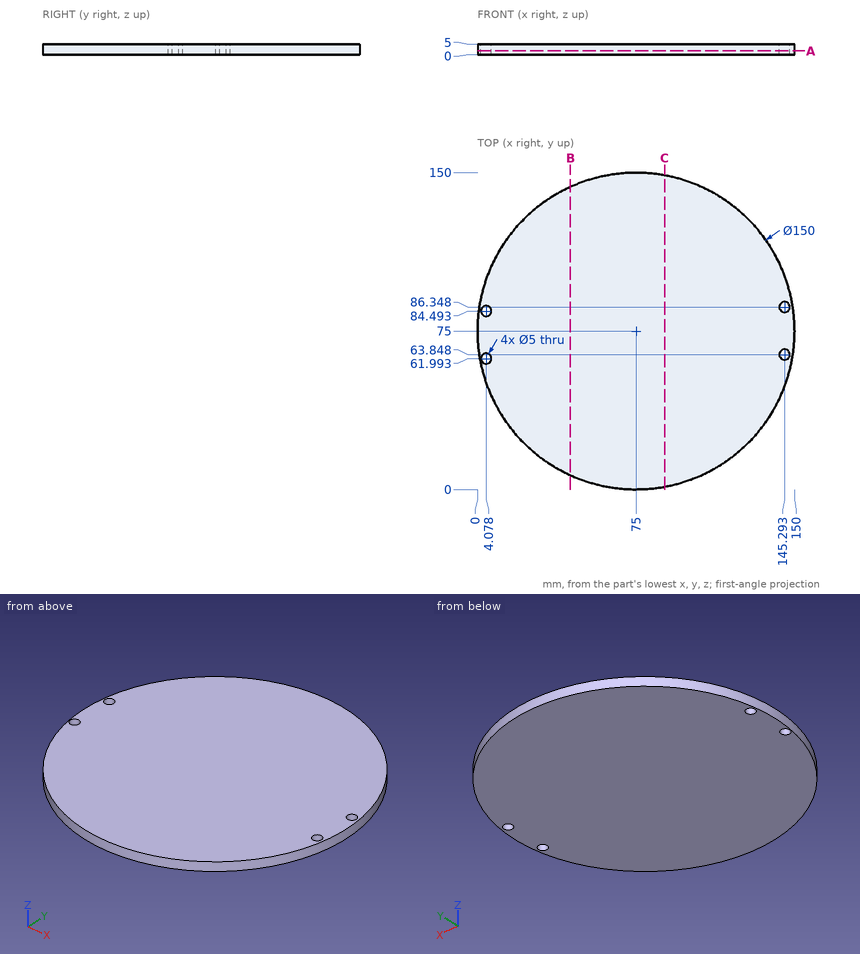
Design review of the part shown in the three views and the two pictorial views. Dimensions are in mm from the part's minimum x, y and z. Give positions to 0.01 mm unless a question says otherwise; leave off trailing zeros. Loops run counter-clockwise (first coordinate to the right, second up) from the corner with the lowest first, then second, coordinate; pieces in that order, holes last. Notation, with made-up numbers: M 35.25,-14.5 L 72.25,-14.5 A26 cw 72.25,14.5 Z; hole C 22,-33.5 d2. An arc over 180 degrees is marked long. Answer as a JSON object with one key per item and string values. Group by question number.
Q1. For probe 1 along X at (y, z) = (85, 1.95) (1 decimal); probe 2 along X at (y, z) = (85.5, 1.75) (1 decimal); probe 3 along Y at (x, z) = (65, 2.8), list the stretches that pass through material, from the lowest coordinate up. Write a range as [from, to].
Q2. Add section C-C on x = 88.5. Give the boundary of the cut face in (y, z) (1 decimal).
Q3. Add section A-A on z = 1.7. Give the boundary of the cut face in (x, y).
Q4. Add section B-B on x = 44. Give the boundary of the cut face in (y, z).
Q5. Insertion check: P1, Ø6, axis at x = 4.08, y = 84.49, coming from the -Z side; P2, Ø3, axis at y = 129.5, z = 2, coming from the +X side (1 decimal); P3, Ø2, axis at x = 43.5, z = 3, coming from the +Y side; P4, Ø2, axis at x = 21.5, z = 1, coming from the +Y side. Each pin has a flat end and moves straight along its axis. Give the tip position at first contact, or say it passes through.
Checked values:
{
 "1": {"probe 1": "[0.7, 1.6], [6.5, 143.2], [147.4, 149.3]", "probe 2": "[0.7, 1.8], [6.4, 142.9], [147.6, 149.3]", "probe 3": "[0.67, 149.33]"},
 "2": {"outline": "M 1.2,0 L 148.8,0 L 148.8,5 L 1.2,5 Z"},
 "3": {"outline": "C 75,75 d150; hole C 4.08,61.99 d5; hole C 4.08,84.49 d5; hole C 145.29,63.85 d5; hole C 145.29,86.35 d5"},
 "4": {"outline": "M 6.71,0 L 143.29,0 L 143.29,5 L 6.71,5 Z"},
 "5": {"P1": "z = 0", "P2": "x = 128.1", "P3": "y = 143.52", "P4": "y = 128.56"}
}
